Source: CAD feature listing. Evaluate the final solid. Frame: model axes, mm. A direction names the side the tool comes from. Coordinates: 2 decimals unless noted, no trailing zeros. Write each loop counter-clockwise with the first axis right and the second up, starting at its lowest first coordinate (ties: lowest second). Pieces come first, ordered by that corner, then holes. Notation, with made-up numbers: (-26.75, 73.25) -> (-1.75, 73.25) arc R27 ccw to (-1.75, 91.25) -> close; hole circle Ø9 at (7.25, 75.5). An arc over 180 degrees is marked (long way). Write item = value, one per line.
from build123d import *

# Parameters (mm, degrees)
SKETCH1_R                                      = 1
BOSS_EXTRUDE1_DEPTH                            = 3
FILLET1_R                                      = 12.5
BOSS_EXTRUDE2_START                            = -1.6
BOSS_EXTRUDE2_DEPTH                            = 1.6
CSK_FOR_M2_FLAT_HEAD_MACHINE_SCREW1_AT_2_COUNT = 2
CSK_FOR_M2_FLAT_HEAD_MACHINE_SCREW1_AT_2_PITCH = 18
FILLET2_R                                      = 5


with BuildPart() as part:
    # Sketch1 → Boss-Extrude1 (new body)
    with BuildSketch(Plane(origin=(0, 0, 0), x_dir=(1, 0, 0), z_dir=(0, 1, 0))):
        with BuildLine():
            Line((32.352380638, 120.740728286), (25.88190451, 96.592582629))
            ThreePointArc((25.88190451, 96.592582629), (75.00161341, 66.141953296), (99.070883715, 13.6))
            Line((99.070883715, 13.6), (76.236612975, 13.6))
            Line((76.236612975, 13.6), (76.236612975, -13.6))
            Line((76.236612975, -13.6), (99.070883715, -13.6))
            ThreePointArc((99.070883715, -13.6), (75.00161341, -66.141953296), (25.88190451, -96.592582629))
            Line((25.88190451, -96.592582629), (32.352380638, -120.740728286))
            ThreePointArc((32.352380638, -120.740728286), (125, 0), (32.352380638, 120.740728286))
        make_face()
        with BuildLine():
            ThreePointArc((80.650826538, 7.4), (79.236612975, 7.4), (79.236612975, 8.814213562))
            Line((79.236612975, 8.814213562), (79.236612975, 9.185786438))
            ThreePointArc((79.236612975, 9.185786438), (79.236612975, 10.6), (80.650826538, 10.6))
            Line((80.650826538, 10.6), (84.022399413, 10.6))
            ThreePointArc((84.022399413, 10.6), (85.436612975, 10.6), (85.436612975, 9.185786438))
            Line((85.436612975, 9.185786438), (85.436612975, 8.814213562))
            ThreePointArc((85.436612975, 8.814213562), (85.436612975, 7.4), (84.022399413, 7.4))
            Line((84.022399413, 7.4), (80.650826538, 7.4))
        make_face(mode=Mode.SUBTRACT)
        with Locations(Location((89.336612975, 9, 0), (0, 0, 270))):
            Circle(SKETCH1_R, mode=Mode.SUBTRACT)
        with BuildLine():
            ThreePointArc((93.236612975, 9.185786438), (93.236612975, 10.6), (94.650826538, 10.6))
            Line((94.650826538, 10.6), (98.022399413, 10.6))
            ThreePointArc((98.022399413, 10.6), (99.362589189, 10.666977143), (99.56285316, 9.340142972))
            ThreePointArc((99.56285316, 9.340142972), (99.599997793, 8.93534776), (99.635496648, 8.530404901))
            ThreePointArc((99.635496648, 8.530404901), (99.303389883, 7.288169964), (98.022399413, 7.4))
            Line((98.022399413, 7.4), (94.650826538, 7.4))
            ThreePointArc((94.650826538, 7.4), (93.236612975, 7.4), (93.236612975, 8.814213562))
            Line((93.236612975, 8.814213562), (93.236612975, 9.185786438))
        make_face(mode=Mode.SUBTRACT)
        with BuildLine():
            ThreePointArc((98.022399413, -7.4), (99.303389883, -7.288169964), (99.635496648, -8.530404901))
            ThreePointArc((99.635496648, -8.530404901), (99.599997793, -8.93534776), (99.56285316, -9.340142972))
            ThreePointArc((99.56285316, -9.340142972), (99.362589189, -10.666977143), (98.022399413, -10.6))
            Line((98.022399413, -10.6), (94.650826538, -10.6))
            ThreePointArc((94.650826538, -10.6), (93.236612975, -10.6), (93.236612975, -9.185786438))
            Line((93.236612975, -9.185786438), (93.236612975, -8.814213562))
            ThreePointArc((93.236612975, -8.814213562), (93.236612975, -7.4), (94.650826538, -7.4))
            Line((94.650826538, -7.4), (98.022399413, -7.4))
        make_face(mode=Mode.SUBTRACT)
        with Locations(Location((89.336612975, -9, 0), (0, 0, 270))):
            Circle(SKETCH1_R, mode=Mode.SUBTRACT)
        with BuildLine():
            ThreePointArc((85.436612975, -9.185786438), (85.436612975, -10.6), (84.022399413, -10.6))
            Line((84.022399413, -10.6), (80.650826538, -10.6))
            ThreePointArc((80.650826538, -10.6), (79.236612975, -10.6), (79.236612975, -9.185786438))
            Line((79.236612975, -9.185786438), (79.236612975, -8.814213562))
            ThreePointArc((79.236612975, -8.814213562), (79.236612975, -7.4), (80.650826538, -7.4))
            Line((80.650826538, -7.4), (84.022399413, -7.4))
            ThreePointArc((84.022399413, -7.4), (85.436612975, -7.4), (85.436612975, -8.814213562))
            Line((85.436612975, -8.814213562), (85.436612975, -9.185786438))
        make_face(mode=Mode.SUBTRACT)
    extrude(amount=BOSS_EXTRUDE1_DEPTH)

    # Fillet1
    fillet1_edges = [part.edges().sort_by_distance(p)[0] for p in [
        (32.352380638, 1.5, 120.740728286),
        (25.88190451, 1.5, 96.592582629),
        (32.352380638, 1.5, -120.740728286),
        (25.88190451, 1.5, -96.592582629),
    ]]
    fillet(fillet1_edges, radius=FILLET1_R - 0.0001)  # a hair under: the kernel refuses the full size

    # Sketch2 → Boss-Extrude2 (add)
    with BuildSketch(Plane(origin=(0, 3, 0), x_dir=(1, 0, 0), z_dir=(0, 1, 0)).offset(BOSS_EXTRUDE2_START)):
        with BuildLine():
            Line((80.650826538, 7.4), (84.022399413, 7.4))
            ThreePointArc((84.022399413, 7.4), (85.436612975, 7.4), (85.436612975, 8.814213562))
            Line((85.436612975, 8.814213562), (85.436612975, 9.185786438))
            ThreePointArc((85.436612975, 9.185786438), (85.436612975, 10.6), (84.022399413, 10.6))
            Line((84.022399413, 10.6), (80.650826538, 10.6))
            ThreePointArc((80.650826538, 10.6), (79.236612975, 10.6), (79.236612975, 9.185786438))
            Line((79.236612975, 9.185786438), (79.236612975, 8.814213562))
            ThreePointArc((79.236612975, 8.814213562), (79.236612975, 7.4), (80.650826538, 7.4))
        make_face()
        with BuildLine():
            Line((93.236612975, 9.185786438), (93.236612975, 8.814213562))
            ThreePointArc((93.236612975, 8.814213562), (93.236612975, 7.4), (94.650826538, 7.4))
            Line((94.650826538, 7.4), (98.022399413, 7.4))
            ThreePointArc((98.022399413, 7.4), (99.303389883, 7.288169964), (99.635496648, 8.530404901))
            ThreePointArc((99.635496648, 8.530404901), (99.599997793, 8.93534776), (99.56285316, 9.340142972))
            ThreePointArc((99.56285316, 9.340142972), (99.362589189, 10.666977143), (98.022399413, 10.6))
            Line((98.022399413, 10.6), (94.650826538, 10.6))
            ThreePointArc((94.650826538, 10.6), (93.236612975, 10.6), (93.236612975, 9.185786438))
        make_face()
        with BuildLine():
            Line((84.022399413, -7.4), (80.650826538, -7.4))
            ThreePointArc((80.650826538, -7.4), (79.236612975, -7.4), (79.236612975, -8.814213562))
            Line((79.236612975, -8.814213562), (79.236612975, -9.185786438))
            ThreePointArc((79.236612975, -9.185786438), (79.236612975, -10.6), (80.650826538, -10.6))
            Line((80.650826538, -10.6), (84.022399413, -10.6))
            ThreePointArc((84.022399413, -10.6), (85.436612975, -10.6), (85.436612975, -9.185786438))
            Line((85.436612975, -9.185786438), (85.436612975, -8.814213562))
            ThreePointArc((85.436612975, -8.814213562), (85.436612975, -7.4), (84.022399413, -7.4))
        make_face()
        with BuildLine():
            Line((93.236612975, -8.814213562), (93.236612975, -9.185786438))
            ThreePointArc((93.236612975, -9.185786438), (93.236612975, -10.6), (94.650826538, -10.6))
            Line((94.650826538, -10.6), (98.022399413, -10.6))
            ThreePointArc((98.022399413, -10.6), (99.362589189, -10.666977143), (99.56285316, -9.340142972))
            ThreePointArc((99.56285316, -9.340142972), (99.599997793, -8.93534776), (99.635496648, -8.530404901))
            ThreePointArc((99.635496648, -8.530404901), (99.303389883, -7.288169964), (98.022399413, -7.4))
            Line((98.022399413, -7.4), (94.650826538, -7.4))
            ThreePointArc((94.650826538, -7.4), (93.236612975, -7.4), (93.236612975, -8.814213562))
        make_face()
    extrude(amount=BOSS_EXTRUDE2_DEPTH)

    # Sketch4 → CSK for M2 Flat Head Machine Screw1 (revolve, cut)
    with BuildSketch(Plane(origin=(89.336612975, 3, -9), x_dir=(0, 0, 1), z_dir=(1, 0, 0))):
        Polygon((0, 0), (0, 3), (1, 3), (1, 1.2), (2, 0.2), (2, 0), align=None)
    csk_for_m2_flat_head_machine_screw1 = revolve(axis=Axis((89.336612975, 9.35, -9), (0, -1, 0)), mode=Mode.SUBTRACT)

    # CSK for M2 Flat Head Machine Screw1 at 2: CSK for M2 Flat Head Machine Screw1 ×2
    with Locations(*[(0, 0, i * CSK_FOR_M2_FLAT_HEAD_MACHINE_SCREW1_AT_2_PITCH) for i in range(1, CSK_FOR_M2_FLAT_HEAD_MACHINE_SCREW1_AT_2_COUNT)]):
        add(csk_for_m2_flat_head_machine_screw1, mode=Mode.SUBTRACT)

    # Fillet2
    fillet2_edges = [part.edges().sort_by_distance(p)[0] for p in [
        (99.070883715, 1.5, -13.6),
        (99.070883715, 1.5, 13.6),
        (76.236612975, 1.5, 13.6),
        (76.236612975, 1.5, -13.6),
    ]]
    fillet(fillet2_edges, radius=FILLET2_R)


solid = part.part
1) Material intervals for probe 1 along X at (y, z) = (2.8, 9); probe 2 along Z at (x, y) = (40, 1.2); probe 3 along Z at (x, y) = (44, 2.8), sorted ascending. Write a range as [from, to].
Answer block:
probe_1 = [76.25, 87.34], [91.34, 124.68]
probe_2 = [-117.22, -91.65], [91.65, 117.22]
probe_3 = [-116.9, -89.8], [89.8, 116.9]
2) Cut plane B-B, the plane y = 2.25. Give the number of separate pieces and of enclosed holes in the cut face, and give its area (3 significant figures).
Answer block:
separate_pieces = 1
enclosed_holes = 2
area = 7,860 mm2
3) First-contact query: pin 1 Ø3 at (x, z) = (89.34, -9) entering from +Y; pin 2 Ø0.7 at (x, y) = (82, 1) entering from +Z; pin 3 Ø1.1 at (x, y) = (82.5, 0.5) entering from -Z. Flat tips, straight axial feed; report the tip coordinate or a pass-through.
Answer block:
pin_1 = 2.3
pin_2 = 94.65
pin_3 = -94.39
4) Cut plane A-A, the plane x = 71. Output: boundary loops of the cut face in (y, z).
Answer block:
outline = (0, -102.88) -> (3, -102.88) -> (3, -70.42) -> (0, -70.42) -> close; (0, 70.42) -> (3, 70.42) -> (3, 102.88) -> (0, 102.88) -> close
5) Pull-direction query (X, two-part tool) for faces 3 (the conical face through (90, 2, -10)), 4 (the flat face through (87, 0, -2)), 5 (the cylindrical face through (77.662, 1.521, 12.096)); classes: +X half, -X half, draft (parallel to the pull), parting line (faces both ways), or undercut.
Answer block:
face_3 = undercut
face_4 = draft
face_5 = -X half
6) Cut plane C-C, the plane x = 49. Output: boundary loops of the cut face in (y, z).
Answer block:
outline = (0, -115) -> (3, -115) -> (3, -87.17) -> (0, -87.17) -> close; (0, 87.17) -> (3, 87.17) -> (3, 115) -> (0, 115) -> close
7) Cut plane D-D, the plane z = -42. Output: boundary loops of the cut face in (x, y), and give its area (3 significant figures).
Answer block:
outline = (90.75, 0) -> (117.73, 0) -> (117.73, 3) -> (90.75, 3) -> close
area = 80.9 mm2
8) Reachability of faces 1 (the cylindrical face through (77.74, 1.521, -12.174)), 2 (the cylindrical face through (124.982, 1.479, 2.096)) from +Z, -Z, +X, -X, +Y, -Y: full face, straight path, thin tool, end or side. Return the list, or none.
Answer block:
face_1 = -X, +Y, -Y
face_2 = +X, +Y, -Y
